Check sheet for the drawn part. Datum: minimum x, y, z corner. Units: mm. A direction names the side the tool comes from. Give positions to 0.01 mm unless a question says otherwise; leave off trailing zeros. Write each loop counter-clockwise with the first axis right and the second up, starting at its lowest first coordinate (ties: lowest second). Pieces come first, ordered by that corner, then holes. Notation, with made-up numbers: (33, 78.5) -> (51, 78.5) arc R17 cw to (51, 99.5) -> close; hole circle Ø4 at (-19, 21.25). An arc over 180 degrees is marked (long way). Write item = value, one per line. Start each with the question number.
1. Cross-section at C-C, the plane x = 14. Record the cut outline in (y, z).
2. Cross-section at D-D, the plane y = 13.75. Record the cut outline in (x, z).
3. Depth check by flat-ended pin: P1, Ø1, axis at x = 22.5, z = 9, coming from the +Y side; P2, Ø1, axis at x = 13, y = 3, coming from the +Z side. Enter the tip coordinate at first touch or a pass-through.
4. Thickness scan on line 1 along X through (y, z) = (0.4, 5.5); line 2 along Z through (x, y) = (20.5, 0.35); line 3 along Y through (x, z) = (4, 2.25). Record the ranges inside material, lowest first.
5. Set-up check for the marked faces 1 and 2: record each of +Z, -Z, +X, -X, +Y, -Y from which the full face is reachable in a straight line by a thin tool's end or side.
6. Cross-section at B-B, the plane z = 5.5. Record the cut outline in (x, y).
7. Cross-section at A-A, the plane x = 20.5. Record the cut outline in (y, z), plus the area to 3 significant figures.
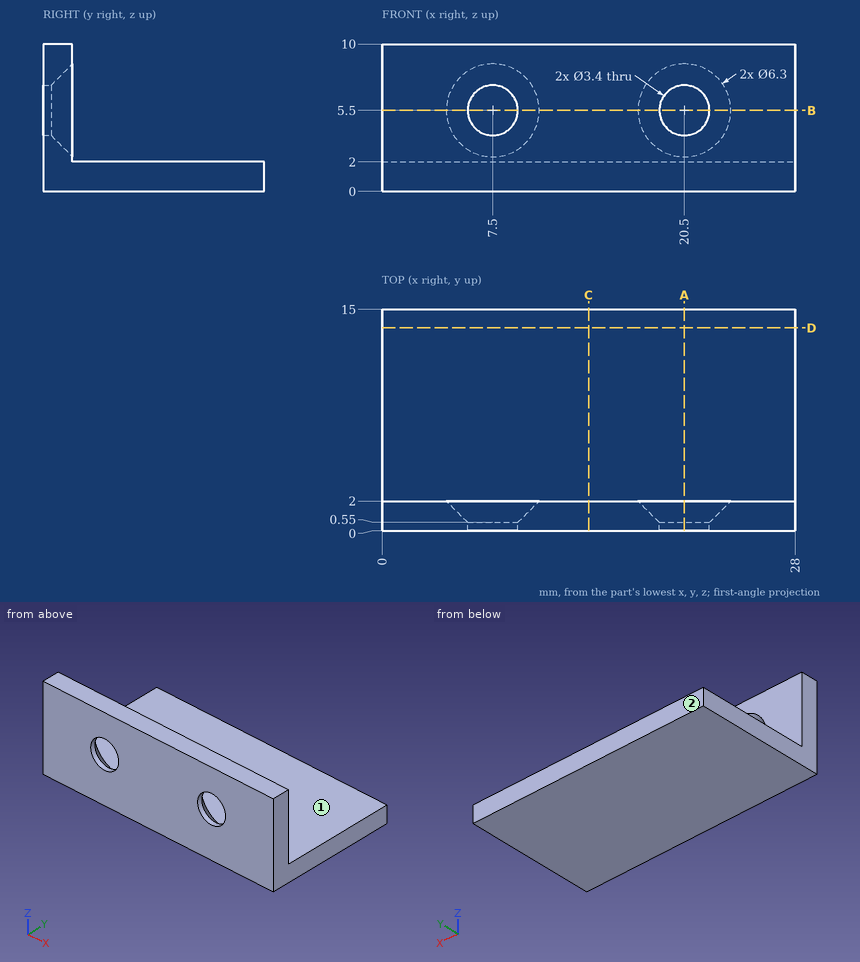
Answers:
q1.outline = (0, 0) -> (15, 0) -> (15, 2) -> (2, 2) -> (2, 10) -> (0, 10) -> close
q2.outline = (0, 0) -> (28, 0) -> (28, 2) -> (0, 2) -> close
q3.P1 = 2
q3.P2 = 2
q4.line_1 = 0 to 5.8, 9.2 to 18.8, 22.2 to 28
q4.line_2 = 0 to 3.8, 7.2 to 10
q4.line_3 = 0 to 2
q5.face_1 = +Z, +X, -X, +Y
q5.face_2 = +Z, -Z, +X, -X, +Y
q6.outline = (0, 0) -> (5.8, 0) -> (5.8, 0.55) -> (4.35, 2) -> (0, 2) -> close; (9.2, 0) -> (18.8, 0) -> (18.8, 0.55) -> (17.35, 2) -> (10.65, 2) -> (9.2, 0.55) -> close; (22.2, 0) -> (28, 0) -> (28, 2) -> (23.65, 2) -> (22.2, 0.55) -> close
q7.outline = (0, 0) -> (15, 0) -> (15, 2) -> (2, 2) -> (2, 2.35) -> (0.55, 3.8) -> (0, 3.8) -> close; (0, 7.2) -> (0.55, 7.2) -> (2, 8.65) -> (2, 10) -> (0, 10) -> close
q7.area = 37.1 mm^2
